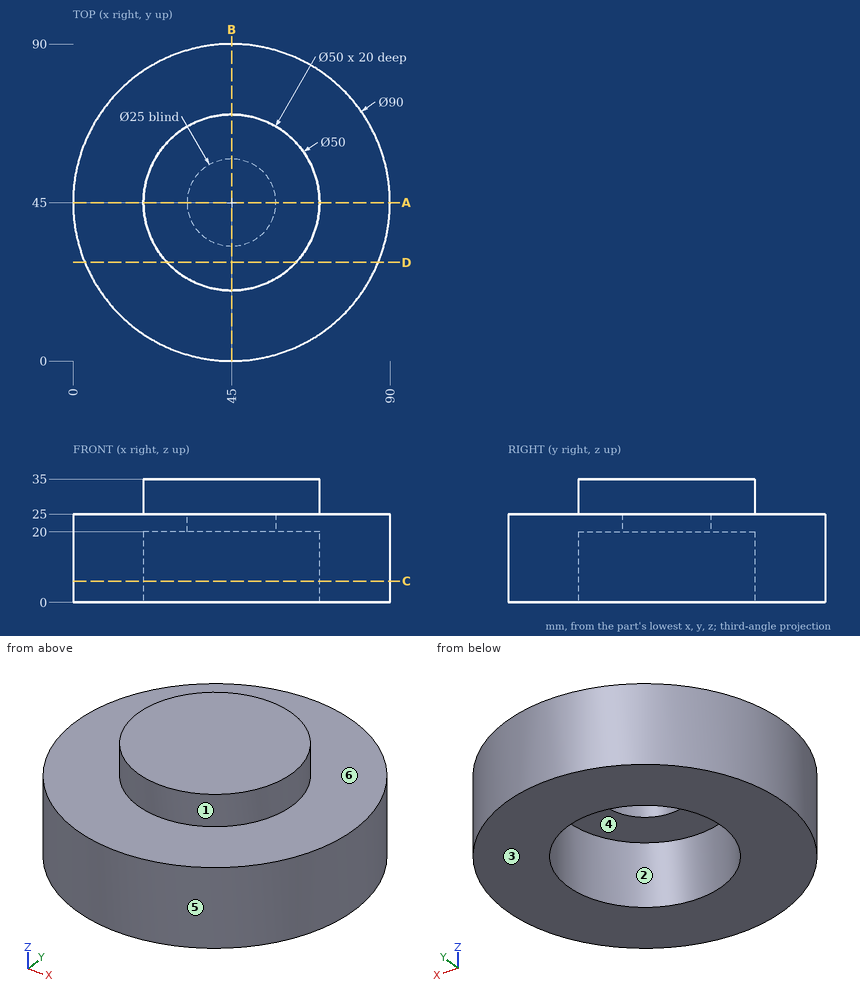
Study the drawing (mm; zero at the part's minimum x, y, z) and answer. A direction names the side the tool comes from. Give positions to 0.01 mm unless a question says otherwise; leave off trailing zeros. Write each loop counter-clockwise with the first axis right and the second up, starting at its lowest first coordinate (ties: lowest second). Pieces come first, ordered by that corner, then holes. Notation, with made-up numbers: (-28.5, 60) - (-7.5, 60) arc R19 cw to (-7.5, 77) - close; hole circle Ø9 at (-7.75, 8). An arc over 180 degrees is marked (long way). Write item = value, one per line. Start each with the question number.
Item 1: Find the intervals of material crossed by probe 1 along Y at (x, z) = (45, 23.8); probe 2 along Y at (x, z) = (45, 14); probe 3 along Z at (x, y) = (56.5, 68.5), in increasing order. Write a range as [from, to].
Item 2: Find section D-D (y = 28). Give the vertices of the cut face in (x, z), then the cut area to 3 significant figures.
Item 3: The mould has two halves that part along X. Classify the marked faces 1, 2, 3 and 4: +X half, -X half, draft (parallel to the pull), parting line (faces both ways), or undercut.
Item 4: Find section A-A (y = 45). Give the vertices of the cut face in (x, z).
Item 5: A tool of negligible diameter and unlimited length cuts with its end or side. For the marked faces 5 and 6, from which of +Z, -Z, +X, -X, +Y, -Y can it reach the whole face along a straight path? Write none if from no direction.
Item 6: Each of these flat-tipped pins is pushed along its axis until it touches: P1, Ø1.5, axis at y = 60.5, z = 26.5, coming from the +X side; P2, Ø2, axis at x = 56.5, z = 6, coming from the -Y side; P3, Ø3, axis at y = 14, z = 8.5, coming from the +X side. Where does it stop, or does it pass through?
Item 7: Find section C-C (z = 6). Give the vertices of the cut face in (x, y), then the cut area to 3 significant figures.
Response:
q1.probe_1 = [0, 32.5], [57.5, 90]
q1.probe_2 = [0, 20], [70, 90]
q1.probe_3 = [0, 25]
q2.outline = (3.33, 0) - (26.67, 0) - (26.67, 20) - (63.33, 20) - (63.33, 0) - (86.67, 0) - (86.67, 25) - (63.33, 25) - (63.33, 35) - (26.67, 35) - (26.67, 25) - (3.33, 25) - close
q2.area = 1,720 mm²
q3.face_1 = parting line
q3.face_2 = undercut
q3.face_3 = draft
q3.face_4 = undercut
q4.outline = (0, 0) - (20, 0) - (20, 20) - (32.5, 20) - (32.5, 25) - (57.5, 25) - (57.5, 20) - (70, 20) - (70, 0) - (90, 0) - (90, 25) - (70, 25) - (70, 35) - (20, 35) - (20, 25) - (0, 25) - close
q5.face_5 = +Z, -Z
q5.face_6 = +Z
q6.P1 = 65.19
q6.P2 = 1.24
q6.P3 = 78.98
q7.outline = circle Ø90 at (45, 45); hole circle Ø50 at (45, 45)
q7.area = 4,400 mm²
